```python
from build123d import *

# Parameters (mm, degrees)
BOSS_EXTRUDE1_DEPTH = 15
SKETCH2_R           = 5.095
CUT_EXTRUDE1_DEPTH  = 10.79
BOSS_EXTRUDE3_START = 15
BOSS_EXTRUDE3_DEPTH = 15
CUT_EXTRUDE2_REACH  = 26.037
SKETCH7_R           = 1.625
CHAMFER2_SIZE       = 2.18
CHAMFER2_SIZE_2     = 3.775870761


with BuildPart() as part:
    # Sketch1 → Boss-Extrude1 (new body)
    with BuildSketch(Plane.XY):
        with BuildLine():
            Line((-3.55, 8.4), (3.55, 8.4))
            ThreePointArc((3.55, 8.4), (6.979467889, 6.979467889), (8.4, 3.55))
            Line((8.4, 3.55), (8.4, -3.55))
            ThreePointArc((8.4, -3.55), (6.979467889, -6.979467889), (3.55, -8.4))
            Line((3.55, -8.4), (-3.55, -8.4))
            ThreePointArc((-3.55, -8.4), (-6.979467889, -6.979467889), (-8.4, -3.55))
            Line((-8.4, -3.55), (-8.4, 3.55))
            ThreePointArc((-8.4, 3.55), (-6.979467889, 6.979467889), (-3.55, 8.4))
        make_face()
    extrude(amount=BOSS_EXTRUDE1_DEPTH)

    # Sketch2 → Cut-Extrude1 (cut)
    with BuildSketch(Plane.XY.offset(15)):
        Circle(SKETCH2_R)
        with BuildLine():
            Line((0.49, 5.071382947), (0.49, 8.4))
            Line((0.49, 8.4), (-0.49, 8.4))
            Line((-0.49, 8.4), (-0.49, 5.071382947))
            ThreePointArc((-0.49, 5.071382947), (0, 5.095), (0.49, 5.071382947))
        make_face()
        with BuildLine():
            Line((5.071382947, -0.49), (8.4, -0.49))
            Line((8.4, -0.49), (8.4, 0.49))
            Line((8.4, 0.49), (5.071382947, 0.49))
            ThreePointArc((5.071382947, 0.49), (5.095, 0), (5.071382947, -0.49))
        make_face()
        with BuildLine():
            Line((-0.49, -5.071382947), (-0.49, -8.4))
            Line((-0.49, -8.4), (0.49, -8.4))
            Line((0.49, -8.4), (0.49, -5.071382947))
            ThreePointArc((0.49, -5.071382947), (0, -5.095), (-0.49, -5.071382947))
        make_face()
        with BuildLine():
            Line((-5.071382947, 0.49), (-8.4, 0.49))
            Line((-8.4, 0.49), (-8.4, -0.49))
            Line((-8.4, -0.49), (-5.071382947, -0.49))
            ThreePointArc((-5.071382947, -0.49), (-5.095, 0), (-5.071382947, 0.49))
        make_face()
    extrude(amount=-CUT_EXTRUDE1_DEPTH, mode=Mode.SUBTRACT)

    # Sketch4 → Boss-Extrude3 (add)
    with BuildSketch(Plane(origin=(0, 0, 0), x_dir=(-1, 0, 0), z_dir=(0, 0, -1)).offset(BOSS_EXTRUDE3_START)):
        with BuildLine():
            Line((-8.4, 3.55), (-8.4, -8.4))
            Line((-8.4, -8.4), (-4, -8.4))
            Line((-4, -8.4), (-4, 4.9))
            Line((-4, 4.9), (4, 4.9))
            Line((4, 4.9), (4, -8.4))
            Line((4, -8.4), (8.4, -8.4))
            Line((8.4, -8.4), (8.4, 3.55))
            ThreePointArc((8.4, 3.55), (6.979467889, 6.979467889), (3.55, 8.4))
            Line((3.55, 8.4), (-3.55, 8.4))
            ThreePointArc((-3.55, 8.4), (-6.979467889, 6.979467889), (-8.4, 3.55))
        make_face()
    extrude(amount=-BOSS_EXTRUDE3_DEPTH)

    # Cut-Extrude2: up to this face of the body (flat: up to its plane)
    cut_extrude2_end = Plane(part.part.faces().sort_by_distance((-8.4, -1.579649264, -2.351915361))[0])
    # Sketch7 → Cut-Extrude2 (cut, up to the picked face)
    with BuildSketch(Plane(origin=(8.4, 0, 0), x_dir=(0, 0, -1), z_dir=(1, 0, 0)), mode=Mode.PRIVATE) as cut_extrude2_sk1:
        with Locations((11.5, -5.175)):
            Circle(SKETCH7_R)
    cut_extrude2_tool1 = split(extrude(cut_extrude2_sk1.sketch, amount=-CUT_EXTRUDE2_REACH, mode=Mode.PRIVATE), bisect_by=cut_extrude2_end, keep=Keep.BOTH, mode=Mode.PRIVATE)
    add(cut_extrude2_tool1.solids().sort_by(Axis((8.4, -5.175, -11.5), (-1, 0, 0)))[0], mode=Mode.SUBTRACT)

    # Chamfer2
    # the kernel refuses this chamfer: 3.775870761, 2.18 mm, written as the material it adds along each edge
    with BuildSketch(Plane(origin=(-3.55, -3.55, 0), x_dir=(0.9389857690160399, 0.343955993675581, 0), z_dir=(-0.343955993675581, 0.9389857690160399, 0))) as chamfer2_piece_1_section:
        Polygon((4.85 + CHAMFER2_SIZE, 0), (4.85, -CHAMFER2_SIZE_2), (4.85, 0), align=None)
    chamfer2_piece_1 = revolve(axis=Axis((-3.55, -3.55, 0), (0, 0, -1)), revolution_arc=315.559918018, mode=Mode.PRIVATE)
    chamfer2_piece_1 = split(chamfer2_piece_1, bisect_by=Plane(origin=(-4, -7.19796441, 1.47894359), z_dir=(-1, 0, 0)), keep=Keep.TOP, mode=Mode.PRIVATE)
    chamfer2_piece_1 = split(chamfer2_piece_1, bisect_by=Plane(origin=(-7.201843372, -8.4, 1.47894359), z_dir=(0, 1, 0)), keep=Keep.TOP, mode=Mode.PRIVATE)
    chamfer2_piece_1 = split(chamfer2_piece_1, bisect_by=Plane(origin=(-8.4, -7.19796441, 1.47894359), z_dir=(1, 0, 0)), keep=Keep.TOP, mode=Mode.PRIVATE)
    add(chamfer2_piece_1)
    with BuildSketch(Plane(origin=(3.55, -3.55, 0), x_dir=(-0.42959466391895607, 0.9030218295990186, 0), z_dir=(-0.9030218295990186, -0.42959466391895607, 0))) as chamfer2_piece_2_section:
        Polygon((4.85, -CHAMFER2_SIZE_2), (4.85 + CHAMFER2_SIZE, 0), (4.85, 0), align=None)
    chamfer2_piece_2 = revolve(axis=Axis((3.55, -3.55, 0), (0, 0, -1)), revolution_arc=315.559918018, mode=Mode.PRIVATE)
    chamfer2_piece_2 = split(chamfer2_piece_2, bisect_by=Plane(origin=(8.4, -7.197964411, 1.478943589), z_dir=(-1, 0, 0)), keep=Keep.TOP, mode=Mode.PRIVATE)
    chamfer2_piece_2 = split(chamfer2_piece_2, bisect_by=Plane(origin=(7.201843372, -8.4, 1.478943589), z_dir=(0, 1, 0)), keep=Keep.TOP, mode=Mode.PRIVATE)
    chamfer2_piece_2 = split(chamfer2_piece_2, bisect_by=Plane(origin=(4, -7.197964411, 1.478943589), z_dir=(1, 0, 0)), keep=Keep.TOP, mode=Mode.PRIVATE)
    add(chamfer2_piece_2)


solid = part.part
```
CAD build for the part. Positions are in the model's coordinates, mm. A direction names the side the tool comes from. Round coordinates to 2 decimals unless told otherwise and drop trailing zeros. Order: outer loops, then holes, each group sorted by start corner. A loop starts at its lowest first (then second) coordinate and runs counter-clockwise, first axis right, second up. Notation, with made-up numbers: (75, 75) - (93, 75) arc R15 cw to (93, 92) - close; hole circle Ø6 at (8.25, -27). An arc over 180 degrees is marked (long way). Use CSV: the item, a comma, the result in double quotes. Start each with the question number.
1) Saw through at D-D (y = 4). List the corners of the cut face in (x, z).
2) Pin check, flat tips, straight feed: pin 1 Ø3.5 at (y, z) = (-5.175, -11.5) entering from -X; pin 2 Ø1.7 at (x, z) = (6, 11.5) entering from -Y; pin 3 Ø1 at (y, z) = (6, 12) entering from -X; pin 4 Ø3 at (x, y) = (0, 2.5) entering from +Z. Stop position of each tip, or through.
3) Two-plate mould, pull along X, no slides. Class faces 5 (the flat face through (7, -0.49, 10)), 6 (the flat face through (-8.4, -1, -4)), 7 (the cylindrical face through (-3.637, -3.568, 9.681)): pulls with the +X half, pulls with the -X half, needs draft (parallel to the pull), parting line crosses it, or undercut.
4) Saw through at C-C (x = 3). List the corners of the cut face in (y, z).
5) Saw through at B-B (z = -5). List the corners of the cut face in (x, y).
6) Wall check: L1, parallel to X at y = -4.5, z = -2.5; L2, parallel to Z at x = -3.25, y = -0.5; L3, parallel to X at y = -6, z = 10. Give the ranges that are in metal, low to high. Write a range as [from, to].
7) Saw through at A-A (z = -11.5). List the corners of the cut face in (x, y).
8) Tool access for faces 1 (the flat face through (0.49, -7, 10)), 2 (the flat face through (0, -2, 0)), 3 (the flat face through (-7, -0.49, 10)), 4 (the cylindrical face through (3.568, -3.637, 9.681)): list every direction of +Z, -Z, +X, -X, +Y, -Y with a clear straight run to the whole face (end or side of a thin tool).
Values follow:
1,outline,"(-8.38, -15) - (-4, -15) - (-4, 0) - (4, 0) - (4, -15) - (8.38, -15) - (8.38, 15) - (3.16, 15) - (3.16, 4.21) - (-3.16, 4.21) - (-3.16, 15) - (-8.38, 15) - close"
2,pin 1,"stops at x = -8.4"
2,pin 2,"stops at y = -8.13"
2,pin 3,"stops at x = -7.99"
2,pin 4,"stops at z = 4.21"
3,face 5,"needs draft"
3,face 6,"pulls with the -X half"
3,face 7,"undercut"
4,outline,"(-8.4, 0) - (4.9, 0) - (4.9, -15) - (8.4, -15) - (8.4, 15) - (4.12, 15) - (4.12, 4.21) - (-4.12, 4.21) - (-4.12, 15) - (-8.4, 15) - close"
5,outline,"(-8.4, -8.4) - (-4, -8.4) - (-4, 4.9) - (4, 4.9) - (4, -8.4) - (8.4, -8.4) - (8.4, 3.55) arc R4.85 ccw to (3.55, 8.4) - (-3.55, 8.4) arc R4.85 ccw to (-8.4, 3.55) - close"
6,L1,"x = [-8.4, -4], [4, 8.4]"
6,L2,"z = [0, 4.21]"
6,L3,"x = [-7.74, -0.49], [0.49, 7.74]"
7,outline,"(-8.4, -8.4) - (-4, -8.4) - (-4, -6.8) - (-8.4, -6.8) - close; (-8.4, -3.55) - (-4, -3.55) - (-4, 4.9) - (4, 4.9) - (4, -3.55) - (8.4, -3.55) - (8.4, 3.55) arc R4.85 ccw to (3.55, 8.4) - (-3.55, 8.4) arc R4.85 ccw to (-8.4, 3.55) - close; (4, -8.4) - (8.4, -8.4) - (8.4, -6.8) - (4, -6.8) - close"
8,face 1,"+Z, +Y, -Y"
8,face 2,"-Z, -Y"
8,face 3,"+Z, +X, -X"
8,face 4,"+Z"
